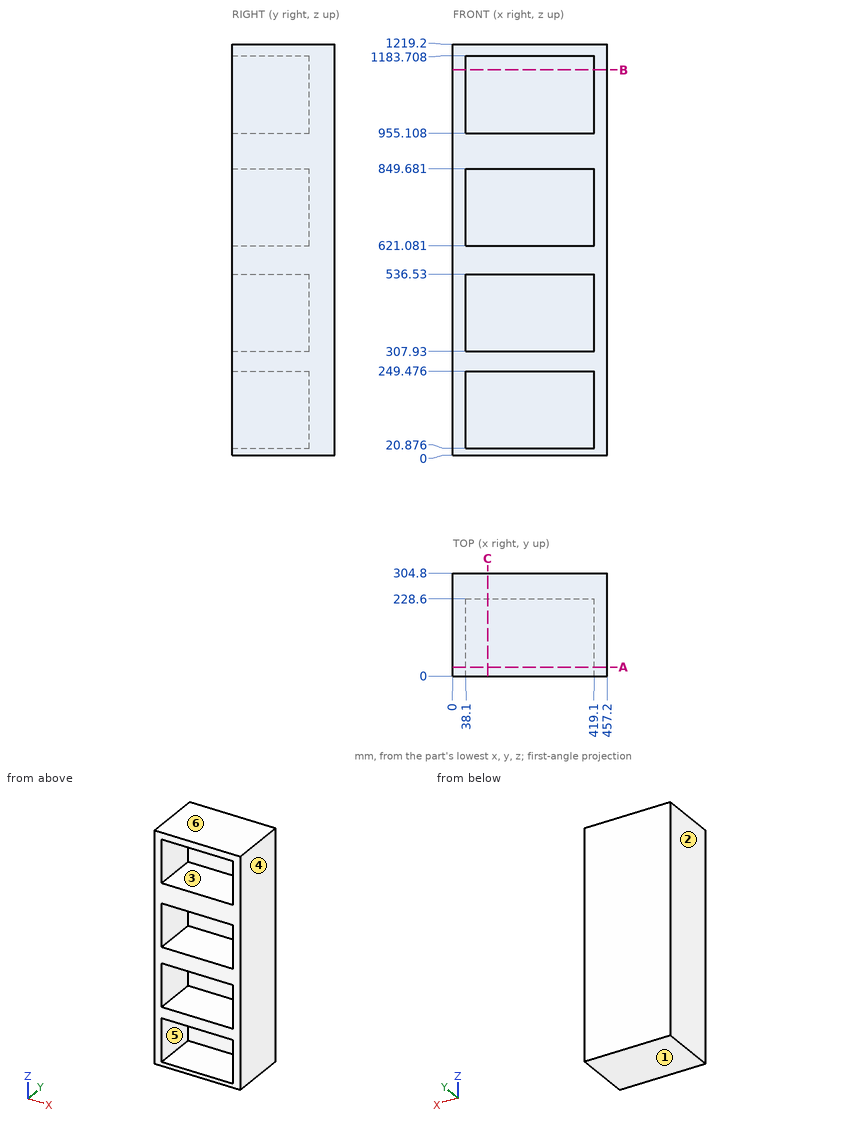
Could you check a few things on this drawing? It's one solid part, dimensions in mm from its lowest x, y, z. A direction names the side the tool comes from. Give positions to 0.01 mm unless a question says otherwise; leave off trailing zeros. Write each loop counter-clockwise with the first axis right and the second up, starting at its lowest first coordinate (ties: lowest second). Pieces come first, ordered by that corner, then holes.
(1) Imagine slicing it at C-C, the plane x = 103.5. Write out the boundary of the cut face in (y, z) (1 decimal).
Output values:
outline: (0, 0) - (304.8, 0) - (304.8, 1219.2) - (0, 1219.2) - (0, 1183.7) - (228.6, 1183.7) - (228.6, 955.1) - (0, 955.1) - (0, 849.7) - (228.6, 849.7) - (228.6, 621.1) - (0, 621.1) - (0, 536.5) - (228.6, 536.5) - (228.6, 307.9) - (0, 307.9) - (0, 249.5) - (228.6, 249.5) - (228.6, 20.9) - (0, 20.9) - close
(2) On a 3-axis mill with a long thin cutter (end or side, diameter ignored), from which of +Z, -Z, +X, -X, +Y, -Y can I reach the whole of each face in a straight line? I mean the marked faces 5 and 6. Say none if no direction works.
Output values:
face 5: -Y
face 6: +Z, +X, -X, +Y, -Y
(3) Will these pins go through, and if not, where does the flat tip stop? pin 1 (5 mm diameter, centred on x = 180, z = 331.5, fed in from -Y); pin 2 (6 mm diameter, centred on x = 330.5, y = 133.5, fed in from -Z).
Output values:
pin 1: stops at y = 228.6
pin 2: stops at z = 0
(4) If I drill on L1, parallel to Z at x = 277.5, y = 209.5 (1 decimal); L2, parallel to X at y = 20, z = 240; L3, parallel to Y at x = 111, z = 179, over which ranges is the centre line in solid material (lowest first)?
Output values:
L1: z = 0 to 20.9, 249.5 to 307.9, 536.5 to 621.1, 849.7 to 955.1, 1183.7 to 1219.2
L2: x = 0 to 38.1, 419.1 to 457.2
L3: y = 228.6 to 304.8
(5) Imagine slicing it at B-B, the plane z = 1142.5. Write out the boundary of the cut face in (x, y), and give its area (3 significant figures).
Output values:
outline: (0, 0) - (38.1, 0) - (38.1, 228.6) - (419.1, 228.6) - (419.1, 0) - (457.2, 0) - (457.2, 304.8) - (0, 304.8) - close
area: 52,300 mm2
(6) Imagine slicing it at A-A, the plane y = 26.5. Write out the boundary of the cut face in (x, z) (1 decimal), and give its area (3 significant figures).
Output values:
outline: (0, 0) - (457.2, 0) - (457.2, 1219.2) - (0, 1219.2) - close; hole (38.1, 20.9) - (419.1, 20.9) - (419.1, 249.5) - (38.1, 249.5) - close; hole (38.1, 307.9) - (419.1, 307.9) - (419.1, 536.5) - (38.1, 536.5) - close; hole (38.1, 621.1) - (419.1, 621.1) - (419.1, 849.7) - (38.1, 849.7) - close; hole (38.1, 955.1) - (419.1, 955.1) - (419.1, 1183.7) - (38.1, 1183.7) - close
area: 209,000 mm2
(7) Thinking about a two-plate mould opening in X: for the marked faces 1, 2, 3 and 4, which applies, pulls with the +X half, pulls with the -X half, needs draft (parallel to the pull), parting line crosses it, or undercut?
Output values:
face 1: needs draft
face 2: pulls with the -X half
face 3: undercut
face 4: pulls with the +X half
